from build123d import *

# Parameters (mm, degrees)
SKETCH_1_W        = 60
SKETCH_1_H        = 90
EXTRUDE_1_DEPTH   = 2
CHAMFER_1_SIZE    = 2
HOLE_WIZARD_M61_D = 6.6


with BuildPart() as part:
    # Эскиз1 → Бобышка-Вытянуть1 (new body)
    with BuildSketch(Plane.XY):
        Rectangle(SKETCH_1_W, SKETCH_1_H)
    extrude(amount=EXTRUDE_1_DEPTH)

    # Фаска1
    chamfer_1_edges = [part.edges().sort_by_distance(p)[0] for p in [
        (30, -45, 1),
        (-30, -45, 1),
        (-30, 45, 1),
        (30, 45, 1),
    ]]
    chamfer(chamfer_1_edges, length=CHAMFER_1_SIZE)

    # Отверстие с зазором M61 (through all)
    with Locations(Plane.XY.offset(2)):
        with Locations((-15, 30), (15, 30), (15, 0), (-15, 0), (-15, -30), (15, -30)):
            Hole(HOLE_WIZARD_M61_D / 2)


solid = part.part
The listing builds one solid part. Answer for the finished solid, in the listing's coordinates (mm). Coordinates: 2 decimals unless noted, no trailing zeros. Write each loop counter-clockwise with the first axis right and the second up, starting at its lowest first coordinate (ties: lowest second). Pieces come first, ordered by that corner, then holes. Notation, with made-up numbers: (-8, 15.5) - (13, 15.5) arc R21 ccw to (13, 33.5) - close; hole circle Ø8 at (67.25, 60.25). An arc over 180 degrees is marked (long way). Put each result on its own line as item: value.
1. A flat-ended cylindrical pin translates along its axis: pin 1 Ø5.5 at (x, y) = (-15, 30) entering from -Z. Find the tip coordinate at first contact, or state that the pin passes through.
Answer sheet:
pin 1: passes through
2. Determine the mould class of faces 1 (the face through (0, 1, 2)), 2 (the face through (-29, -44, 1)), 3 (the face through (18.3, 30.1, 1)) for opening direction Y: pulls with the +Y half, pulls with the -Y half, needs draft (parallel to the pull), parting line crosses it, or undercut.
Answer sheet:
face 1: needs draft
face 2: pulls with the -Y half
face 3: undercut
3. The part is cut by section C-C on z = 0.8. Give the vertices of the cut face in (x, y).
Answer sheet:
outline: (-30, -43) - (-28, -45) - (28, -45) - (30, -43) - (30, 43) - (28, 45) - (-28, 45) - (-30, 43) - close; hole circle Ø6.6 at (-15, -30); hole circle Ø6.6 at (-15, 0); hole circle Ø6.6 at (-15, 30); hole circle Ø6.6 at (15, -30); hole circle Ø6.6 at (15, 0); hole circle Ø6.6 at (15, 30)
4. The part is cut by section D-D on y = -2. Give the vertices of the cut face in (x, z).
Answer sheet:
outline: (-30, 0) - (-17.62, 0) - (-17.62, 2) - (-30, 2) - close; (-12.38, 0) - (12.38, 0) - (12.38, 2) - (-12.38, 2) - close; (17.62, 0) - (30, 0) - (30, 2) - (17.62, 2) - close
5. The part is cut by section A-A on x = -15. Give the vertices of the cut face in (y, z).
Answer sheet:
outline: (-45, 0) - (-33.3, 0) - (-33.3, 2) - (-45, 2) - close; (-26.7, 0) - (-3.3, 0) - (-3.3, 2) - (-26.7, 2) - close; (3.3, 0) - (26.7, 0) - (26.7, 2) - (3.3, 2) - close; (33.3, 0) - (45, 0) - (45, 2) - (33.3, 2) - close
6. The part is cut by section B-B on y = 30. Give the vertices of the cut face in (x, z).
Answer sheet:
outline: (-30, 0) - (-18.3, 0) - (-18.3, 2) - (-30, 2) - close; (-11.7, 0) - (11.7, 0) - (11.7, 2) - (-11.7, 2) - close; (18.3, 0) - (30, 0) - (30, 2) - (18.3, 2) - close
7. Find the intervals of material crossed by line 1 along Y through (x, z) = (15, 1.25); line 2 along X through (y, z) = (-31, 0.9); line 3 along X through (y, z) = (28.5, 1.6), in increasing order. Write a range as from..to.
Answer sheet:
line 1: y = -45..-33.3, -26.7..-3.3, 3.3..26.7, 33.3..45
line 2: x = -30..-18.14, -11.86..11.86, 18.14..30
line 3: x = -30..-17.94, -12.06..12.06, 17.94..30
